Verification items for the finished model (mm, model axes). A direction names the side the tool comes from. Give positions to 0.01 mm unless a question says otherwise; leave off trailing zeros. Write each loop counter-clockwise with the first axis right and the second up, starting at its lowest first coordinate (ties: lowest second). Pieces come first, ordered by that corner, then holes. Notation, with made-up numbers: M 78.5,10.25 L 98.5,10.25 A9 cw 98.5,20.25 Z; hole C -24.5,-13.75 d3. An arc over 180 degrees is marked long. Answer as a JSON object with one key per item and string values.
```python
from build123d import *

# Parameters (mm, degrees)
SKETCH1_R           = 139
BOSS_EXTRUDE5_DEPTH = 220
CHAMFER6_SIZE       = 20
SKETCH9_R           = 119
BOSS_EXTRUDE6_DEPTH = 20
BOSS_EXTRUDE7_START = 20
SKETCH10_R          = 10
BOSS_EXTRUDE7_DEPTH = 20


with BuildPart() as part:
    # Sketch1 → Boss-Extrude5 (new body)
    with BuildSketch(Plane(origin=(0, 0, 0), x_dir=(1, 0, 0), z_dir=(0, 1, 0))):
        with Locations(Location((0, 0, 0), (0, 0, 270))):
            Circle(SKETCH1_R)
    extrude(amount=BOSS_EXTRUDE5_DEPTH)

    # Chamfer6
    chamfer6_edges = [part.edges().sort_by_distance(p)[0] for p in [
        (0, 220, -139),
    ]]
    chamfer(chamfer6_edges, length=CHAMFER6_SIZE)

    # Sketch9 → Boss-Extrude6 (add)
    with BuildSketch(Plane(origin=(0, 220, 0), x_dir=(1, 0, 0), z_dir=(0, 1, 0))):
        with Locations(Location((0, 0, 0), (0, 0, 270))):
            Circle(SKETCH9_R)
    extrude(amount=BOSS_EXTRUDE6_DEPTH)

    # Sketch10 → Boss-Extrude7 (add)
    # profile 1 of 20: a face of its own
    with BuildSketch(Plane.XZ.offset(BOSS_EXTRUDE7_START)):
        with BuildLine():
            ThreePointArc((-139, 0), (-98.287842585, 98.287842585), (0, 139))
            Line((0, 139), (-139, 139))
            Line((-139, 139), (-139, 0))
        make_face()
        with Locations(Location((-122.899316497, 122.899316497, 0), (0, 0, 270))):
            Circle(SKETCH10_R, mode=Mode.SUBTRACT)
    # profile 2 of 20: a face of its own
    with BuildSketch(Plane.XZ.offset(BOSS_EXTRUDE7_START)):
        with BuildLine():
            Line((139, 139), (0, 139))
            ThreePointArc((0, 139), (98.287842585, 98.287842585), (139, 0))
            Line((139, 0), (139, 139))
        make_face()
        with Locations(Location((122.899316497, 122.899316497, 0), (0, 0, 270))):
            Circle(SKETCH10_R, mode=Mode.SUBTRACT)
    # profile 3 of 20: a face of its own
    with BuildSketch(Plane.XZ.offset(BOSS_EXTRUDE7_START)):
        with BuildLine():
            Line((139, -139), (139, 0))
            ThreePointArc((139, 0), (98.287842585, -98.287842585), (0, -139))
            Line((0, -139), (139, -139))
        make_face()
        with Locations(Location((122.899316497, -122.899316497, 0), (0, 0, 270))):
            Circle(SKETCH10_R, mode=Mode.SUBTRACT)
    # profile 4 of 20: a face of its own
    with BuildSketch(Plane.XZ.offset(BOSS_EXTRUDE7_START)):
        with BuildLine():
            ThreePointArc((0, -139), (-98.287842585, -98.287842585), (-139, 0))
            Line((-139, 0), (-139, -139))
            Line((-139, -139), (0, -139))
        make_face()
        with Locations(Location((-122.899316497, -122.899316497, 0), (0, 0, 270))):
            Circle(SKETCH10_R, mode=Mode.SUBTRACT)
    # profile 5 of 20: a face of its own
    with BuildSketch(Plane.XZ.offset(BOSS_EXTRUDE7_START)):
        with BuildLine():
            ThreePointArc((139, 0), (98.287842585, 98.287842585), (0, 139))
            Line((0, 139), (0, 0))
            Line((0, 0), (139, 0))
        make_face()
    # profile 6 of 20: a face of its own
    with BuildSketch(Plane.XZ.offset(BOSS_EXTRUDE7_START)):
        with BuildLine():
            Line((0, 0), (0, 139))
            ThreePointArc((0, 139), (-98.287842585, 98.287842585), (-139, 0))
            Line((-139, 0), (0, 0))
        make_face()
    # profile 7 of 20: a face of its own
    with BuildSketch(Plane.XZ.offset(BOSS_EXTRUDE7_START)):
        with BuildLine():
            Line((139, 0), (0, 0))
            Line((0, 0), (0, -139))
            ThreePointArc((0, -139), (98.287842585, -98.287842585), (139, 0))
        make_face()
    # profile 8 of 20: a face of its own
    with BuildSketch(Plane.XZ.offset(BOSS_EXTRUDE7_START)):
        with BuildLine():
            Line((0, -139), (0, 0))
            Line((0, 0), (-139, 0))
            ThreePointArc((-139, 0), (-98.287842585, -98.287842585), (0, -139))
        make_face()
    # profile 9 of 20: a face of its own
    with BuildSketch(Plane.XZ.offset(BOSS_EXTRUDE7_START)):
        with BuildLine():
            ThreePointArc((139, 0), (98.287842585, 98.287842585), (0, 139))
            Line((0, 139), (0, 0))
            Line((0, 0), (139, 0))
        make_face()
    # profile 10 of 20: a face of its own
    with BuildSketch(Plane.XZ.offset(BOSS_EXTRUDE7_START)):
        with BuildLine():
            Line((0, 0), (0, 139))
            ThreePointArc((0, 139), (-98.287842585, 98.287842585), (-139, 0))
            Line((-139, 0), (0, 0))
        make_face()
    # profile 11 of 20: a face of its own
    with BuildSketch(Plane.XZ.offset(BOSS_EXTRUDE7_START)):
        with BuildLine():
            Line((139, 0), (0, 0))
            Line((0, 0), (0, -139))
            ThreePointArc((0, -139), (98.287842585, -98.287842585), (139, 0))
        make_face()
    # profile 12 of 20: a face of its own
    with BuildSketch(Plane.XZ.offset(BOSS_EXTRUDE7_START)):
        with BuildLine():
            Line((0, -139), (0, 0))
            Line((0, 0), (-139, 0))
            ThreePointArc((-139, 0), (-98.287842585, -98.287842585), (0, -139))
        make_face()
    # profile 13 of 20: a face of its own
    with BuildSketch(Plane.XZ.offset(BOSS_EXTRUDE7_START)):
        with BuildLine():
            ThreePointArc((139, 0), (98.287842585, 98.287842585), (0, 139))
            Line((0, 139), (0, 0))
            Line((0, 0), (139, 0))
        make_face()
    # profile 14 of 20: a face of its own
    with BuildSketch(Plane.XZ.offset(BOSS_EXTRUDE7_START)):
        with BuildLine():
            Line((0, 0), (0, 139))
            ThreePointArc((0, 139), (-98.287842585, 98.287842585), (-139, 0))
            Line((-139, 0), (0, 0))
        make_face()
    # profile 15 of 20: a face of its own
    with BuildSketch(Plane.XZ.offset(BOSS_EXTRUDE7_START)):
        with BuildLine():
            Line((139, 0), (0, 0))
            Line((0, 0), (0, -139))
            ThreePointArc((0, -139), (98.287842585, -98.287842585), (139, 0))
        make_face()
    # profile 16 of 20: a face of its own
    with BuildSketch(Plane.XZ.offset(BOSS_EXTRUDE7_START)):
        with BuildLine():
            Line((0, -139), (0, 0))
            Line((0, 0), (-139, 0))
            ThreePointArc((-139, 0), (-98.287842585, -98.287842585), (0, -139))
        make_face()
    # profile 17 of 20: a face of its own
    with BuildSketch(Plane.XZ.offset(BOSS_EXTRUDE7_START)):
        with BuildLine():
            ThreePointArc((139, 0), (98.287842585, 98.287842585), (0, 139))
            Line((0, 139), (0, 0))
            Line((0, 0), (139, 0))
        make_face()
    # profile 18 of 20: a face of its own
    with BuildSketch(Plane.XZ.offset(BOSS_EXTRUDE7_START)):
        with BuildLine():
            Line((0, 0), (0, 139))
            ThreePointArc((0, 139), (-98.287842585, 98.287842585), (-139, 0))
            Line((-139, 0), (0, 0))
        make_face()
    # profile 19 of 20: a face of its own
    with BuildSketch(Plane.XZ.offset(BOSS_EXTRUDE7_START)):
        with BuildLine():
            Line((139, 0), (0, 0))
            Line((0, 0), (0, -139))
            ThreePointArc((0, -139), (98.287842585, -98.287842585), (139, 0))
        make_face()
    # profile 20 of 20: a face of its own
    with BuildSketch(Plane.XZ.offset(BOSS_EXTRUDE7_START)):
        with BuildLine():
            Line((0, -139), (0, 0))
            Line((0, 0), (-139, 0))
            ThreePointArc((-139, 0), (-98.287842585, -98.287842585), (0, -139))
        make_face()
    extrude(amount=-BOSS_EXTRUDE7_DEPTH)


solid = part.part
```
1) Release check for a two-part mould opening along X. For faces 5 (the face through (123.34, -10.14, -112.91)), 6 (the face through (-117.118, 219.029, -26.007)), 7 (the face through (2, 240, -2)) record: pulls with the +X half, pulls with the -X half, needs draft (parallel to the pull), parting line crosses it, or undercut.
Completed:
{"face 5": "undercut", "face 6": "parting line crosses it", "face 7": "needs draft"}
2) Thickness scan on L1, parallel to X at y = 83.5, z = 41; L2, parallel to Y at x = -106.5, z = 113.5; L3, parallel to X at y = 192, z = 32.5. Record the ranges inside material, lowest first.
Completed:
{"L1": "x = -132.82 to 132.82", "L2": "y = -20 to 0", "L3": "x = -135.15 to 135.15"}
3) Section check A-A on y = 192. Record the boundary of the cut face in (x, z), and give its area (3 significant figures).
Completed:
{"outline": "C 0,0 d278", "area": "60,700 mm2"}
4) Go/stop test with flat-tipped pins: pin 1 (8 mm diameter, centred on x = -92.5, y = 29.5, fed in from -Z); pin 2 (4 mm diameter, centred on y = 37.5, z = 11, fed in from +X); pin 3 (4 mm diameter, centred on x = 73.5, y = 34, fed in from -Z); pin 4 (18 mm diameter, centred on x = 122.9, z = -122.9, fed in from +Y). Record where each tip stops, or that it passes through.
Completed:
{"pin 1": "stops at z = -107.19", "pin 2": "stops at x = 138.71", "pin 3": "stops at z = -119.2", "pin 4": "passes through"}
5) Access from +Z, -Z, +X, -X, +Y, -Y to the whole of each face (thin tool, end or side, straight path). Record for faces 1 (the face through (-106, 0, -110)), 2 (the face through (117.987, 229.86, -15.491)), 3 (the face through (105, 0, 106)), 4 (the face through (105, 0, -110)).
Completed:
{"face 1": "-Z, -X, +Y", "face 2": "+Y", "face 3": "+Z, +X, +Y", "face 4": "-Z, +X, +Y"}
